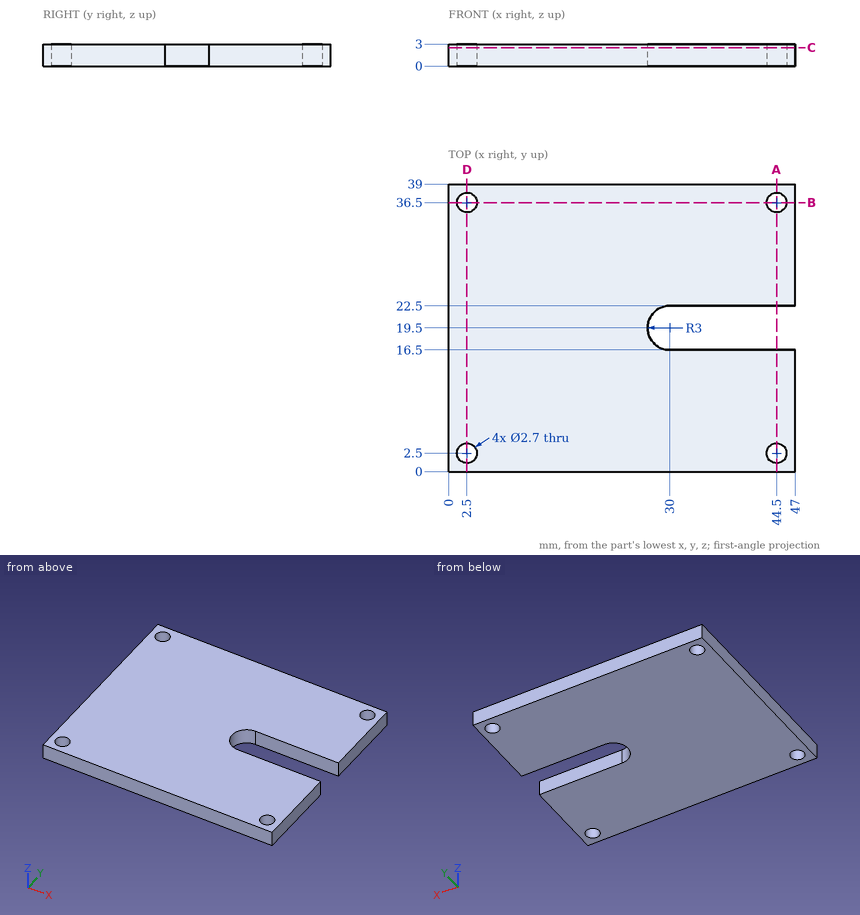
Drawing for the job (mm, zero at the part's lowest x, y, z). Round coordinates to 2 decimals unless told otherwise and drop trailing zeros. Write each loop counter-clockwise with the first axis right and the second up, starting at its lowest first coordinate (ties: lowest second). Pieces come first, ordered by that corner, then holes. Notation, with made-up numbers: M 42.5,47 L 74.5,47 A27 ccw 74.5,76 Z; hole C 25,19 d10. An arc over 180 degrees is marked long. One line per question, with ' | ' between items.
1. Cut at D-D on x = 2.5. Write the cut outline in (y, z), and give its area (3 significant figures).
Working result:
outline: M 0,0 L 1.15,0 L 1.15,3 L 0,3 Z; M 3.85,0 L 35.15,0 L 35.15,3 L 3.85,3 Z; M 37.85,0 L 39,0 L 39,3 L 37.85,3 Z | area: 101 mm2
2. Cut at C-C on z = 2.5. Write the cut outline in (x, y), and give its area (3 significant figures).
Working result:
outline: M 0,0 L 47,0 L 47,16.5 L 30,16.5 A3 cw 30,22.5 L 47,22.5 L 47,39 L 0,39 Z; hole C 2.5,2.5 d2.7; hole C 2.5,36.5 d2.7; hole C 44.5,2.5 d2.7; hole C 44.5,36.5 d2.7 | area: 1,690 mm2
3. Cut at A-A on x = 44.5. Write the cut outline in (y, z), and give its area (3 significant figures).
Working result:
outline: M 0,0 L 1.15,0 L 1.15,3 L 0,3 Z; M 3.85,0 L 16.5,0 L 16.5,3 L 3.85,3 Z; M 22.5,0 L 35.15,0 L 35.15,3 L 22.5,3 Z; M 37.85,0 L 39,0 L 39,3 L 37.85,3 Z | area: 82.8 mm2
4. Probe L1, parallel to Y at x = 2.5, z = 1.2; L2, parallel to Y at x = 42, z = 2.65; L3, parallel to Y at x = 44.5, z = 1.5. List the from-to ranges inside material, lowest first. Write a range as from..to.
Working result:
L1: 0..1.15, 3.85..35.15, 37.85..39 | L2: 0..16.5, 22.5..39 | L3: 0..1.15, 3.85..16.5, 22.5..35.15, 37.85..39
5. Cut at B-B on y = 36.5. Write the cut outline in (x, z), and give its area (3 significant figures).
Working result:
outline: M 0,0 L 1.15,0 L 1.15,3 L 0,3 Z; M 3.85,0 L 43.15,0 L 43.15,3 L 3.85,3 Z; M 45.85,0 L 47,0 L 47,3 L 45.85,3 Z | area: 125 mm2
6. Pin check, flat tips, straight feed: pin 1 Ø3 at (x, y) = (44.5, 2.5) entering from +Z; pin 2 Ø1.6 at (x, y) = (2.5, 36.5) entering from -Z. Stop position of each tip, or through.
Working result:
pin 1: z = 3 | pin 2: through
